Autodesk Inventor part; units mm, degrees
ref_plane "YZ Plane" through (0, 0, 0) normal (1, 0, 0) x (0, 1, 0)
ref_plane "XZ Plane" through (0, 0, 0) normal (0, 1, 0) x (-1, 0, 0)
ref_plane "XY Plane" through (0, 0, 0) normal (0, 0, 1) x (1, 0, 0)
sketch "Sketch1" plane through (0, 0, 0) normal (0, 0, 1) x (1, 0, 0)
  line L0 (0, 0) -> (25, 0)
  line L1 (25, 0) -> (25, 6)
  line L2 (25, 6) -> (17.1289, 6)
  arc A0 (14.6584, 10.7019) -> (5.5, 37.729) centre (0, 20.8) ccw
  line L3 (0, 0) -> (0, 8)
  arc A1 (0, 8) -> (0.5, 33.5902) centre (0, 20.8) ccw
  arc A2 (14.6584, 10.7019) -> (17.1289, 6) centre (17.1289, 9) ccw
  line L4 (5.5, 37.729) -> (5.5, 44.729)
  line L5 (5.5, 44.729) -> (0.5, 44.729)
  line L6 (0.5, 44.729) -> (0.5, 33.5902)
  point P0 (9.8894, 6)
  dimension "d0" = 12.8
  dimension "d2" = 5
  dimension "d3" = 25
  dimension "d4" = 6
  dimension "d5" = 8
  dimension "d6" = 3
  dimension "d7" = 1
  dimension "d8" = 5
  dimension "d9" = 7
extrude "Extrusion1" add sketch "Sketch1" along normal blind 15
sketch "Sketch2" plane through (17.1289, 6, 0) normal (0, 1, 0) x (1, 0, 0)
  line L0 (7.8711, 0) -> (7.8711, -15)
  line L1 (7.8711, -15) -> (0, 0) construction
  line L2 (7.8711, 0) -> (0, 0)
  circle A0 centre (3.9355, -7.5) radius 1.6
  point P0 (-17.1289, 0)
  dimension "d15" = 3.2
extrude "Extrusion2" cut sketch "Sketch2" against normal through all
chamfer "Chamfer1" distance 4 angle 45 2 edges at (25, 3, 15) (25, 3, 0)
sketch "Sketch3" plane through (5.5, 37.729, 0) normal (1, 0, 0) x (0, 0, -1)
  line L0 (-15, 0) -> (0, 7) construction
  point P0 (0, -37.729)
  point P1 (-7.5, 3.5)
hole "Hole1" at (5.5, 41.229, 7.5) direction (-1, 0, 0) diameter 3.2 end through all
fillet "Fillet1" radius 3 2 edges at (3, 44.729, 0) (3, 44.729, 15)
fillet "Fillet1" radius 1 2 edges at (5.5, 37.729, 7.5) (0.5, 33.5902, 7.5)
mirror "Mirror1" about plane through (0, 8, 0) normal (-1, 0, 0)
properties part number "atomizer_holder"
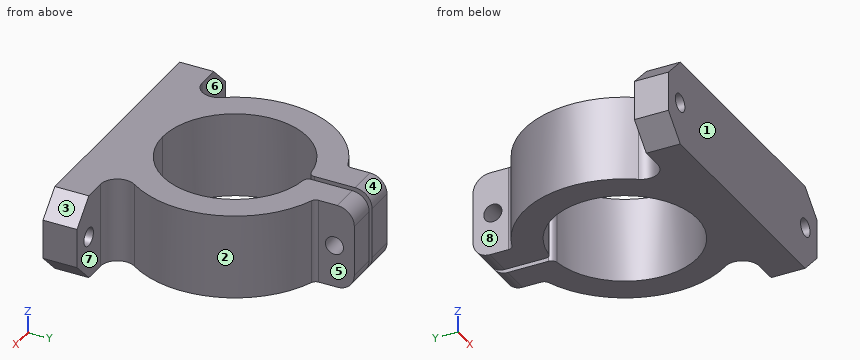
Build history of the part. All positions in model axes, mm. Face numbers are marked on the shaded views. A direction names the side the tool comes from. Round coordinates to 2 decimals unless told otherwise and drop trailing zeros. Write each loop counter-clockwise with the first axis right and the second up, starting at its lowest first coordinate (ties: lowest second). Pieces come first, ordered by that corner, then holes. Notation, with made-up numbers: M -22,11.25 L 8,11.25 A17 ccw 8,30.25 Z; hole C 70.5,29 d1. An arc over 180 degrees is marked long. Use CSV: the item, a comma, the result in double quotes.
1. Wall check: probe 1 along X at (y, z) = (1.85, 7.5); probe 2 along X at (y, z) = (39, 6.25); probe 3 along Y at (x, z) = (-1.95, 7.5). Give the ranges that are in metal, low to high. Write a range as from..to.
Reply:
probe 1,"x = -25..-22.66, -19.46..19.46, 22.66..25"
probe 2,"x = -5.5..-0.5, 0.5..5.5"
probe 3,"y = 0..8.15, 33.45..39.63, 42.83..44.73"
2. Two-plate mould, pull along Y, no slides. Class the marked faces 1, 2, 3 and 4: +Y half, -Y half, draft (parallel to the pull), parting line (faces both ways), or undercut.
Reply:
face 1,"-Y half"
face 2,"undercut"
face 3,"draft"
face 4,"+Y half"
3. Saw through at C-C (z = 14). Give the cut face in (x, y), plus the area to 3 significant figures.
Reply:
outline,"M -22,0 L 22,0 L 22,6 L 17.13,6 A3 cw 14.66,10.7 A17.8 ccw 6.15,37.5 A1 cw 5.5,38.44 L 5.5,43.97 L 0.5,43.97 L 0.5,34.52 A1 ccw 1.39,33.52 A12.8 cw 0,8 A12.8 cw -1.39,33.52 A1 ccw -0.5,34.52 L -0.5,43.97 L -5.5,43.97 L -5.5,38.44 A1 cw -6.15,37.5 A17.8 ccw -14.66,10.7 A3 cw -17.13,6 L -22,6 Z"
area,"775 mm²"
4. Saw through at A-A (x = -9.5). Give the cut face in (y, z), plus the area to 3 significant figures.
Reply:
outline,"M 0,0 L 12.22,0 L 12.22,15 L 0,15 Z; M 29.38,0 L 35.85,0 L 35.85,15 L 29.38,15 Z"
area,"280 mm²"
5. Flat gauge pins, fed straight in: pin 1 (1.9 mm diameter, centred on x = -21.06, z = 7.5, fed in from -Y); pin 2 (7 mm diameter, centred on y = 42.5, z = 10, fed in from -X); pin 3 (5 mm diameter, centred on x = 21.06, z = 7.5, fed in from -Y); pin 4 (4 mm diameter, centred on y = 41.229, z = 7.5, fed in from +X). Where does each tip first touch, or does it go through?
Reply:
pin 1,"passes through"
pin 2,"stops at x = -5.5"
pin 3,"stops at y = 0"
pin 4,"stops at x = 5.5"
6. Tool access for the marked faces 5, 6, 7 and 8: list every direction of +Z, -Z, +X, -X, +Y, -Y with a clear straight run to the whole face (end or side of a thin tool).
Reply:
face 5,"+Z, -Z, +X, +Y"
face 6,"+Z, -Z, -X"
face 7,"+Z, -Z, +X"
face 8,"+Z, -Z, -X, +Y"
7. Saw through at B-B (y = 12.5). Give the cut face in (x, z).
Reply:
outline,"M -15.75,0 L -9.74,0 L -9.74,15 L -15.75,15 Z; M 9.74,0 L 15.75,0 L 15.75,15 L 9.74,15 Z"
8. Saw through at D-D (z = 6.75). State how many separate pieces and enclosed holes the cut face has, plus the area to 3 significant figures.
Reply:
separate pieces,"5"
enclosed holes,"0"
area,"757 mm²"
